Check sheet for the modelled part. Datum: model origin and axes. Units: mm. Coordinates: 2 decimals unless noted, no trailing zeros. Loops run counter-clockwise (first coordinate to the right, second up) from the corner with the lowest first, then second, coordinate; pieces in that order, holes last. Notation, with made-up numbers: M 57.5,29 L 115.5,29 A20 ccw 115.5,56 Z; hole C -10,-24 d1. An arc over 180 degrees is marked long. Use CSV: the item, a comma, the result in double quotes. Start each with the question number.
(1) Section check B-B on x = 46. Record the cut outline in (y, z).
(2) Draft check along X on faces 1 (the flat face through (-1, 0, -5)), 2 (the flat face through (-45, 1, -18)), 3 (the cylindrical face through (-39.086, 0.776, -0.352)). Enter one of: pulls with the +X half, pulls with the -X half, needs draft (parallel to the pull), parting line crosses it, or undercut.
(3) Go/stop test with flat-tipped pins: pin 1 Ø3 at (x, z) = (-37.5, 0) entering from +Y; pin 2 Ø12 at (x, z) = (-16, -18.5) entering from -Y. Record where each tip stops, or that it passes through.
(4) Section check A-A on y = 0.4. Give the number of separate pieces and of enclosed holes in the cut face, and give its area (3 significant figures).
(5) Scan lines: line 1 (Z direction, x = 47.46, y = 1.15); line 2 (X direction, y = 0.5, z = -8.5); line 3 (Z direction, x = 41, y = 1.1). Record each from-to range of solid material in increasing order.
from build123d import *

# Parameters (mm, degrees)
SKETCH1_W             = 110
SKETCH1_H             = 50
BOSS_EXTRUDE1_DEPTH   = 1.53
SKETCH6_W             = 141.050966046
SKETCH6_H             = 69.53153639
SKETCH6_W_2           = 110
SKETCH6_H_2           = 50
CUT_EXTRUDE4_DEPTH    = 62.736058345
SKETCH2_R             = 0.5
PUSHBUTTONHOLES_DEPTH = 62.736058345
SKETCH7_R             = 1.625
MOUNT_HOLES_DEPTH     = 62.736058345
SKETCH5_R             = 0.5
RJ12HOLES_DEPTH       = 62.736058345
LPATTERN1_COUNT       = 3
LPATTERN1_PITCH       = 25
LPATTERN1_COL_COUNT   = 3
LPATTERN1_COL_PITCH   = 25


with BuildPart() as part:
    # Sketch1 → Boss-Extrude1 (new body)
    with BuildSketch(Plane(origin=(0, 0, 0), x_dir=(1, 0, 0), z_dir=(0, 1, 0))):
        with Locations((0, 3)):
            Rectangle(SKETCH1_W, SKETCH1_H)
    extrude(amount=BOSS_EXTRUDE1_DEPTH)

    # Sketch6 → Cut-Extrude4 (cut, through all)
    # profile 1 of 4: a face of its own
    with BuildSketch(Plane(origin=(0, 1.53, 0), x_dir=(1, 0, 0), z_dir=(0, 1, 0))):
        Rectangle(SKETCH6_W, SKETCH6_H)
        with Locations((0, 3)):
            Rectangle(SKETCH6_W_2, SKETCH6_H_2, mode=Mode.SUBTRACT)
    # profile 2 of 4: a face of its own
    with BuildSketch(Plane(origin=(0, 1.53, 0), x_dir=(1, 0, 0), z_dir=(0, 1, 0))):
        Polygon((55, -18), (-55, -18), (-55, -22), (-52, -22), (-28, -22), (55, -22), align=None)
    # profile 3 of 4: a face of its own
    with BuildSketch(Plane(origin=(0, 1.53, 0), x_dir=(1, 0, 0), z_dir=(0, 1, 0))):
        Polygon((-55, 8), (-35, 28), (-55, 28), align=None)
    # profile 4 of 4: a face of its own
    with BuildSketch(Plane(origin=(0, 1.53, 0), x_dir=(1, 0, 0), z_dir=(0, 1, 0))):
        Polygon((55, 28), (35, 28), (55, 8), align=None)
    extrude(amount=-CUT_EXTRUDE4_DEPTH, mode=Mode.SUBTRACT)

    # Sketch2 → PushButtonHoles (cut, through all)
    with BuildSketch(Plane(origin=(0, 1.53, 0), x_dir=(1, 0, 0), z_dir=(0, 1, 0))):
        with Locations(Location((-2.54, -8.46, 0), (0, 0, 270))):
            Circle(SKETCH2_R)
        with Locations(Location((0, -8.46, 0), (0, 0, 270))):
            Circle(SKETCH2_R)
        with Locations(Location((2.54, -8.46, 0), (0, 0, 270))):
            Circle(SKETCH2_R)
        with Locations(Location((-2.54, -13.54, 0), (0, 0, 270))):
            Circle(SKETCH2_R)
        with Locations(Location((0, -13.54, 0), (0, 0, 270))):
            Circle(SKETCH2_R)
        with Locations(Location((2.54, -13.54, 0), (0, 0, 270))):
            Circle(SKETCH2_R)
    pushbuttonholes = extrude(amount=-PUSHBUTTONHOLES_DEPTH, mode=Mode.SUBTRACT)

    # Sketch7 → Mount Holes (cut, through all)
    with BuildSketch(Plane(origin=(0, 1.53, 0), x_dir=(1, 0, 0), z_dir=(0, 1, 0))):
        with Locations(Location((-37.5, 0, 0), (0, 0, 270))):
            Circle(SKETCH7_R)
        with Locations(Location((37.5, 0, 0), (0, 0, 270))):
            Circle(SKETCH7_R)
    extrude(amount=-MOUNT_HOLES_DEPTH, mode=Mode.SUBTRACT)

    # Sketch5 → RJ12Holes (cut, through all)
    with BuildSketch(Plane(origin=(0, 1.53, 0), x_dir=(1, 0, 0), z_dir=(0, 1, 0))):
        with Locations(Location((-2.54, 17.54, 0), (0, 0, 270))):
            Circle(SKETCH5_R)
        with Locations(Location((0, 17.54, 0), (0, 0, 270))):
            Circle(SKETCH5_R)
        with Locations(Location((2.54, 17.54, 0), (0, 0, 270))):
            Circle(SKETCH5_R)
        with Locations(Location((-2.54, 15, 0), (0, 0, 270))):
            Circle(SKETCH5_R)
        with Locations(Location((0, 15, 0), (0, 0, 270))):
            Circle(SKETCH5_R)
        with Locations(Location((2.54, 15, 0), (0, 0, 270))):
            Circle(SKETCH5_R)
    extrude(amount=-RJ12HOLES_DEPTH, mode=Mode.SUBTRACT)

    # LPattern1: PushButtonHoles ×3
    with Locations(*[(i * LPATTERN1_PITCH, 0, 0) for i in range(1, LPATTERN1_COUNT)]):
        add(pushbuttonholes, mode=Mode.SUBTRACT)

    # LPattern1 col: PushButtonHoles ×3
    with Locations(*[(-i * LPATTERN1_COL_PITCH, 0, 0) for i in range(1, LPATTERN1_COL_COUNT)]):
        add(pushbuttonholes, mode=Mode.SUBTRACT)


solid = part.part
Outcome:
1,outline,"M 0,-17 L 1.53,-17 L 1.53,18 L 0,18 Z"
2,face 1,"needs draft"
2,face 2,"pulls with the -X half"
2,face 3,"undercut"
3,pin 1,"passes through"
3,pin 2,"stops at y = 0"
4,separate pieces,"1"
4,enclosed holes,"38"
4,area,"4,620 mm²"
5,line 1,"z = -15.54 to 7.96, 8.96 to 13.04, 14.04 to 18"
5,line 2,"x = -54.5 to 54.5"
5,line 3,"z = -22 to 18"
